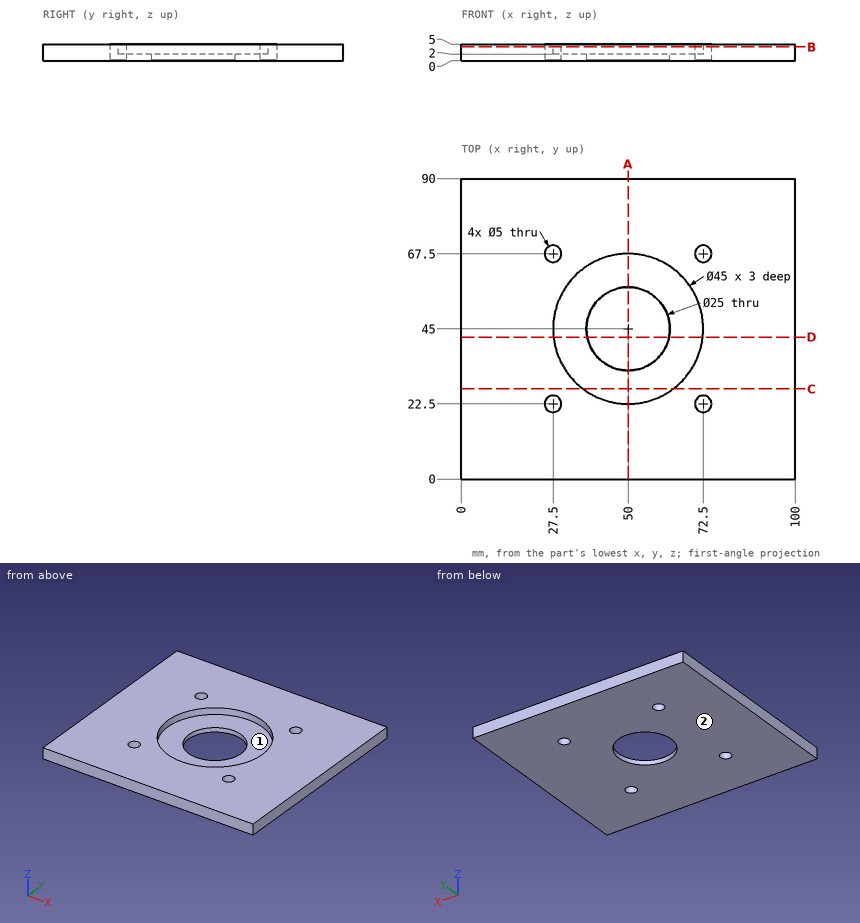
For this review, use the dimensioned drawing (mm, ordinates from the lowest corner) and the shaded views. Round coordinates to 2 decimals unless told otherwise and drop trailing zeros. Loops run counter-clockwise (first coordinate to the right, second up) from the corner with the lowest first, then second, coordinate; pieces in that order, holes last. Notation, with made-up numbers: (33, 4.5) -> (60, 4.5) arc R18 ccw to (60, 17.5) -> close; hole circle Ø3 at (-15.5, 52.5). An arc over 180 degrees is marked (long way). Write item = value, one per line. Start each with the question number.
Item 1: Take a section at D-D on y = 42.5. Give the boundary of the cut face in (x, z), plus the area to 3 significant figures.
Item 2: Insertion check: pin 1 (6 mm diameter, centred on x = 72.5, y = 22.5, fed in from +Z); pin 2 (22.5 mm diameter, centred on x = 56, y = 37.5, fed in from +Z). Each pin has a flat end and moves straight along its axis. Give the tip position at first contact, or say it passes through.
Item 3: To check wall thickness, follow L1, parallel to Y at x = 27.5, z = 1.75; L2, parallel to Y at x = 50, z = 1.35; L3, parallel to X at y = 21.5, z = 2. State the ranges of each line that lie inside material, in increasing order.
Item 4: Mouldability with a two-part tool opening along X and no side actions: class the marked faces 1 and 2 as released by +X, released by -X, zero draft, split by the parting line, or undercut.
Item 5: Take a section at C-C on y = 27. Give the boundary of the cut face in (x, z).
Item 6: Take a section at A-A on x = 50. Give the boundary of the cut face in (y, z).
Item 7: Take a section at B-B on z = 4.15. Give the boundary of the cut face in (x, y).
Result:
q1.outline = (0, 0) -> (37.75, 0) -> (37.75, 2) -> (27.64, 2) -> (27.64, 5) -> (0, 5) -> close; (62.25, 0) -> (100, 0) -> (100, 5) -> (72.36, 5) -> (72.36, 2) -> (62.25, 2) -> close
q1.area = 317 mm²
q2.pin_1 = 5
q2.pin_2 = 2
q3.L1 = 0 to 20, 25 to 65, 70 to 90
q3.L2 = 0 to 32.5, 57.5 to 90
q3.L3 = 0 to 25.21, 29.79 to 70.21, 74.79 to 100
q4.face_1 = undercut
q4.face_2 = zero draft
q5.outline = (0, 0) -> (100, 0) -> (100, 5) -> (63.5, 5) -> (63.5, 2) -> (36.5, 2) -> (36.5, 5) -> (0, 5) -> close
q6.outline = (0, 0) -> (32.5, 0) -> (32.5, 2) -> (22.5, 2) -> (22.5, 5) -> (0, 5) -> close; (57.5, 0) -> (90, 0) -> (90, 5) -> (67.5, 5) -> (67.5, 2) -> (57.5, 2) -> close
q7.outline = (0, 0) -> (100, 0) -> (100, 90) -> (0, 90) -> close; hole circle Ø5 at (27.5, 22.5); hole circle Ø5 at (27.5, 67.5); hole circle Ø45 at (50, 45); hole circle Ø5 at (72.5, 22.5); hole circle Ø5 at (72.5, 67.5)
